```python
from build123d import *

# Parameters (mm, degrees)
F2_DEPTH = 10
F3_R     = 12.5
F4_DEPTH = 5
F7_DEPTH = 2


with BuildPart() as f2:
    # F1 (on face) → F2 (new body)
    with BuildSketch(Plane.XY):
        with BuildLine():
            Line((0, 0), (15, 0))
            ThreePointArc((15, 0), (13.2889854694, 6.9572167707), (8.5462846407, 12.3272470098))
            ThreePointArc((8.5462846407, 12.3272470098), (0.4015789928, 14.9946235135), (-7.8742218987, 12.7670133348))
            Line((-7.8742218987, 12.7670133348), (-9.1641377572, 11.8751243853))
            ThreePointArc((-9.1641377572, 11.8751243853), (-13.4622075894, 6.6158118792), (-15, 0))
            Line((-15, 0), (0, 0))
        make_face()
        with BuildLine():
            ThreePointArc((-15, 0), (0, -15), (15, 0))
            Line((15, 0), (0, 0))
            Line((0, 0), (-15, 0))
        make_face()
    extrude(amount=F2_DEPTH)

    # F3 (on face) → F4 (join)
    with BuildSketch(Plane.XY.offset(10)):
        Circle(F3_R)
    extrude(amount=F4_DEPTH)

    # F5 (on face) → F6 (revolve)
    with BuildSketch(Plane.XY.offset(15)):
        with BuildLine():
            Line((0, -11), (0, 11))
            ThreePointArc((0, 11), (-11, 0), (0, -11))
        make_face()
    revolve(axis=Axis((0, 0, 15), (0, 1, 0)))

    # F0 (on Top) → F7 (join)
    with BuildSketch(Plane.XY):
        with BuildLine():
            ThreePointArc((-9.1641377572, -11.8751243853), (-13.4622075894, -6.6158118792), (-15, 0))
            Line((-15, 0), (-17.0049901825, 0))
            ThreePointArc((-17.0049901825, 0), (-17.9996312672, -1.9911334725), (-20.1890252755, -2.3917296142))
            ThreePointArc((-20.1890252755, -2.3917296142), (-21.0448007649, -2.843869621), (-22, -3))
            Line((-22, -3), (-9.1641377572, -11.8751243853))
        make_face()
        with BuildLine():
            Line((17.25, 0), (15, 0))
            ThreePointArc((15, 0), (13.4622075894, -6.6158118792), (9.1641377572, -11.8751243853))
            Line((9.1641377572, -11.8751243853), (22, -3))
            ThreePointArc((22, -3), (20.9058923217, -2.7933722251), (19.9625, -2.2019522588))
            ThreePointArc((19.9625, -2.2019522588), (18.0819247199, -1.7468722048), (17.25, 0))
        make_face()
        with BuildLine():
            ThreePointArc((21.75, 0), (21.2468722048, -1.4180752801), (19.9625, -2.2019522588))
            ThreePointArc((19.9625, -2.2019522588), (20.9058923217, -2.7933722251), (22, -3))
            ThreePointArc((22, -3), (24.1213203436, -2.1213203436), (25, 0))
            Line((25, 0), (22, 0))
            Line((22, 0), (21.75, 0))
        make_face()
        with BuildLine():
            ThreePointArc((8.5462846407, 12.3272470098), (13.2889854694, 6.9572167707), (15, 0))
            Line((15, 0), (17.25, 0))
            ThreePointArc((17.25, 0), (18.0819247199, 1.7468722048), (19.9625, 2.2019522588))
            ThreePointArc((19.9625, 2.2019522588), (20.9058923217, 2.7933722251), (22, 3))
            Line((22, 3), (8.5462846407, 12.3272470098))
        make_face()
        with BuildLine():
            ThreePointArc((22, 3), (20.9058923217, 2.7933722251), (19.9625, 2.2019522588))
            ThreePointArc((19.9625, 2.2019522588), (21.2468722048, 1.4180752801), (21.75, 0))
            Line((21.75, 0), (22, 0))
            Line((22, 0), (25, 0))
            ThreePointArc((25, 0), (24.1213203436, 2.1213203436), (22, 3))
        make_face()
        with BuildLine():
            Line((-17.0049901825, 0), (-15, 0))
            ThreePointArc((-15, 0), (-13.4622075894, 6.6158118792), (-9.1641377572, 11.8751243853))
            Line((-9.1641377572, 11.8751243853), (-22, 3))
            ThreePointArc((-22, 3), (-21.0448007649, 2.843869621), (-20.1890252755, 2.3917296142))
            ThreePointArc((-20.1890252755, 2.3917296142), (-17.9996312672, 1.9911334725), (-17.0049901825, 0))
        make_face()
        with BuildLine():
            ThreePointArc((-21.9856042642, 0), (-21.4864306958, 1.4956659562), (-20.1890252755, 2.3917296142))
            ThreePointArc((-20.1890252755, 2.3917296142), (-21.0448007649, 2.843869621), (-22, 3))
            ThreePointArc((-22, 3), (-24.1213203436, 2.1213203436), (-25, 0))
            Line((-25, 0), (-22, 0))
            Line((-22, 0), (-21.9856042642, 0))
        make_face()
        with BuildLine():
            ThreePointArc((-22, -3), (-21.0448007649, -2.843869621), (-20.1890252755, -2.3917296142))
            ThreePointArc((-20.1890252755, -2.3917296142), (-21.4864306958, -1.4956659562), (-21.9856042642, 0))
            Line((-21.9856042642, 0), (-22, 0))
            Line((-22, 0), (-25, 0))
            ThreePointArc((-25, 0), (-24.1213203436, -2.1213203436), (-22, -3))
        make_face()
    extrude(amount=F7_DEPTH)


solid = f2.part
```
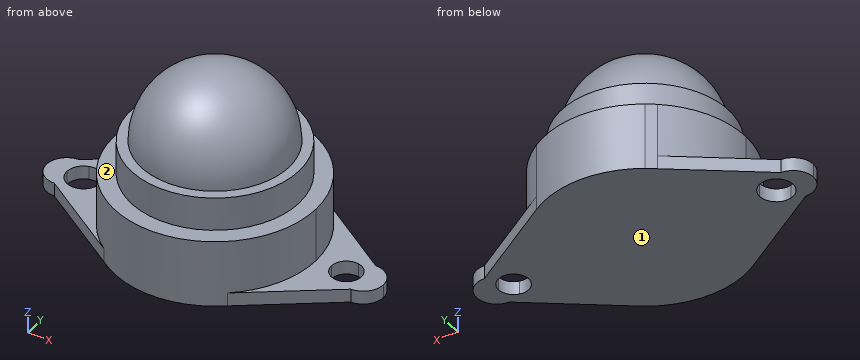
Verification items for the finished model (mm, model axes). Face numbers are marked on the shaded views. A direction names the side the tool comes from. Coordinates: 2 decimals unless noted, no trailing zeros. Loops run counter-clockwise (first coordinate to the right, second up) from the corner with the lowest first, then second, coordinate; pieces in that order, holes last. Notation, with made-up numbers: (-14.75, 56) -> (36.25, 56) arc R11 cw to (36.25, 64) -> close; hole circle Ø2 at (49, 79). An arc over 180 degrees is marked (long way). Put each result on its own line as item: value.
1. Section check D-D, the plane y = -8. Record the boundary of the cut face in (x, z), then the cut area to 3 significant figures.
Result set:
outline: (-14.77, 0) -> (14.77, 0) -> (14.77, 2) -> (12.69, 2) -> (12.69, 10) -> (9.6, 10) -> (9.6, 15) -> (7.55, 15) arc R7.55 ccw to (-7.55, 15) -> (-9.6, 15) -> (-9.6, 10) -> (-12.69, 10) -> (-12.69, 2) -> (-14.77, 2) -> close
area: 448 mm^2
2. Tool access check on the marked faces 1 and 2. Record the directions out of +Z, -Z, +X, -X, +Y, -Y that give a thin tool (end or side, any length) a straight path to the whole face; none if there is none.
Result set:
face 1: -Z, +X, -X, +Y, -Y
face 2: +Z
3. Section check C-C, the plane y = 6.75. Record the boundary of the cut face in (x, z), then the cut area to 3 significant figures.
Result set:
outline: (-16.58, 0) -> (16.59, 0) -> (16.59, 2) -> (13.4, 2) -> (13.4, 10) -> (10.52, 10) -> (10.52, 15) -> (8.69, 15) arc R8.69 ccw to (-8.69, 15) -> (-10.52, 15) -> (-10.52, 10) -> (-13.4, 10) -> (-13.4, 2) -> (-16.58, 2) -> close
area: 504 mm^2
4. Section check B-B, the plane x = 0. Record the boundary of the cut face in (y, z), then the cut area to 3 significant figures.
Result set:
outline: (-15, 0) -> (15, 0) -> (15, 10) -> (12.5, 10) -> (12.5, 15) -> (11, 15) arc R11 ccw to (-11, 15) -> (-12.5, 15) -> (-12.5, 10) -> (-15, 10) -> close
area: 615 mm^2
5. Thickness scan on line 1 (Z direction, x = 12.5, y = 5.25); line 2 (Z direction, x = 0, y = 0); line 3 (Y direction, x = -8, z = 1.5). Record the ranges inside material, lowest first.
Result set:
line 1: z = 0 to 10
line 2: z = 0 to 26
line 3: y = -12.69 to 12.68
6. Gauge pin test, flat ends, axial feed: P1, Ø1, axis at y = 8.5, z = 16, coming from the -X side; P2, Ø5, axis at x = -1.5, y = -4.5, coming from the -Z side; P3, Ø6, axis at y = 4, z = 5.5, coming from the +X side; P4, Ø5, axis at y = 2.5, z = 13, coming from the +X side. Record the tip position at first contact, or that the pin passes through.
Result set:
P1: stops at x = -7.49
P2: stops at z = 0
P3: stops at x = 14.97
P4: stops at x = 12.5
7. Section check A-A, the plane z = 4.5. Record the boundary of the cut face in (x, y).
Result set:
outline: (-9.16, 11.88) arc R15 ccw (long way) to (-7.87, 12.77) -> close
